Source: CAD feature listing. Evaluate the final solid. Frame: model axes, mm. A direction names the side the tool comes from. Give positions to 0.01 mm unless a question says otherwise; leave off trailing zeros. Loops run counter-clockwise (first coordinate to the right, second up) from the corner with the lowest first, then second, coordinate; pieces in that order, holes last. Notation, with made-up numbers: M -12,45 L 10,45 A10 ccw 10,64 Z; hole C 34,-5 d11. An arc over 180 degrees is marked long. Put each result on its own line as item: value.
from build123d import *

# Parameters (mm, degrees)
SKETCH1_R           = 5.969
SKETCH1_R_2         = 4.572
BASE_EXTRUDE_DEPTH  = 13.97
BOSS_EXTRUDE1_DEPTH = 7.112
SKETCH3_W           = 4.826
SKETCH3_H           = 3.048
CUT_EXTRUDE1_DEPTH  = 1.524
CUT_EXTRUDE2_START  = -6.605477
SKETCH4_W           = 1.524
SKETCH4_H           = 4.064
CUT_EXTRUDE2_DEPTH  = 6.605477
CUT_EXTRUDE3_REACH  = 10.382
SKETCH5_R           = 0.8001
BOSS_EXTRUDE2_DEPTH = 1.524
SKETCH7_R           = 0.508
CUT_EXTRUDE4_DEPTH  = 10.144
BOSS_EXTRUDE3_DEPTH = 1.524
BOSS_EXTRUDE4_START = -3.048
BOSS_EXTRUDE4_DEPTH = 3.048
CUT_EXTRUDE5_START  = -1.1176
CUT_EXTRUDE5_DEPTH  = 1.1176
CUT_EXTRUDE6_DEPTH  = 4.064


with BuildPart() as part:
    # Sketch1 → Base-Extrude (new body)
    with BuildSketch(Plane.XY):
        Circle(SKETCH1_R)
        Circle(SKETCH1_R_2, mode=Mode.SUBTRACT)
    extrude(amount=BASE_EXTRUDE_DEPTH)

    # Sketch2 → Boss-Extrude1 (add)
    with BuildSketch(Plane.XY.offset(13.5636)):
        with BuildLine():
            Line((-2.413, -5.459523056), (-3.937, -8.763))
            Line((-3.937, -8.763), (-3.937, -12.065))
            Line((-3.937, -12.065), (-2.413, -12.065))
            Line((-2.413, -12.065), (-2.413, -15.113))
            Line((-2.413, -15.113), (2.413, -15.113))
            Line((2.413, -15.113), (2.413, -12.065))
            Line((2.413, -12.065), (3.937, -12.065))
            Line((3.937, -12.065), (3.937, -8.763))
            Line((3.937, -8.763), (2.413, -5.459523056))
            ThreePointArc((2.413, -5.459523056), (0, -5.969), (-2.413, -5.459523056))
        make_face()
    extrude(amount=-BOSS_EXTRUDE1_DEPTH)

    # Sketch3 → Cut-Extrude1 (cut)
    with BuildSketch(Plane.XY.offset(13.97)):
        with Locations((0, -13.589)):
            Rectangle(SKETCH3_W, SKETCH3_H)
    extrude(amount=-CUT_EXTRUDE1_DEPTH, mode=Mode.SUBTRACT)

    # Sketch4 → Cut-Extrude2 (cut)
    with BuildSketch(Plane.XZ.offset(12.065).offset(CUT_EXTRUDE2_START)):
        with Locations((3.175, 8.4836)):
            Rectangle(SKETCH4_W, SKETCH4_H)
        with Locations((-3.175, 8.4836)):
            Rectangle(SKETCH4_W, SKETCH4_H)
    extrude(amount=CUT_EXTRUDE2_DEPTH, mode=Mode.SUBTRACT)

    # Sketch5 → Cut-Extrude3 (cut, up to next)
    with BuildSketch(Plane(origin=(2.413, 0, 0), x_dir=(0, 0, -1), z_dir=(1, 0, 0)), mode=Mode.PRIVATE) as cut_extrude3_sk1:
        with Locations((-9.7155, -10.577465123)):
            Circle(SKETCH5_R)
    cut_extrude3_tool1 = extrude(cut_extrude3_sk1.sketch, amount=-CUT_EXTRUDE3_REACH, mode=Mode.PRIVATE) & part.part
    add(cut_extrude3_tool1.solids().sort_by_distance((2.413, -10.577465, 9.7155))[0], mode=Mode.SUBTRACT)

    # Sketch6 → Boss-Extrude2 (add)
    with BuildSketch(Plane.XY.offset(9.144)):
        with BuildLine():
            Line((-2.794, 5.274706153), (-1.524, 12.451775059))
            ThreePointArc((-1.524, 12.451775059), (-1.263283995, 12.902874385), (-0.773656889, 13.081))
            Line((-0.773656889, 13.081), (0.773656889, 13.081))
            ThreePointArc((0.773656889, 13.081), (1.263283995, 12.902874385), (1.524, 12.451775059))
            Line((1.524, 12.451775059), (2.794, 5.274706153))
            ThreePointArc((2.794, 5.274706153), (0, 5.969), (-2.794, 5.274706153))
        make_face()
    extrude(amount=-BOSS_EXTRUDE2_DEPTH)

    # Sketch7 → Cut-Extrude4 (cut, through all)
    with BuildSketch(Plane.XY.offset(9.144)):
        with Locations((0, 11.811)):
            Circle(SKETCH7_R)
    extrude(amount=-CUT_EXTRUDE4_DEPTH, mode=Mode.SUBTRACT)

    # Sketch8 → Boss-Extrude3 (add)
    with BuildSketch(Plane(origin=(0, 0, 0), x_dir=(-1, 0, 0), z_dir=(0, 0, -1))):
        with BuildLine():
            Line((-1.016, 4.873623966), (-1.016, 5.881896378))
            ThreePointArc((-1.016, 5.881896378), (0, 5.969), (1.016, 5.881896378))
            Line((1.016, 5.881896378), (1.016, 4.873623966))
            ThreePointArc((1.016, 4.873623966), (0, 4.9784), (-1.016, 4.873623966))
        make_face()
    extrude(amount=BOSS_EXTRUDE3_DEPTH)

    # Sketch9 → Boss-Extrude4 (add)
    with BuildSketch(Plane.XZ.offset(15.113).offset(BOSS_EXTRUDE4_START)):
        Polygon((2.413, 9.4996), (2.9718, 8.7376), (2.9718, 7.2136), (2.413, 6.4516), align=None)
        Polygon((-2.413, 9.4996), (-2.9718, 8.7376), (-2.9718, 7.2136), (-2.413, 6.4516), align=None)
    extrude(amount=BOSS_EXTRUDE4_DEPTH)

    # Sketch10 → Cut-Extrude5 (cut)
    with BuildSketch(Plane.XY.offset(13.5636).offset(CUT_EXTRUDE5_START)):
        with BuildLine():
            Line((-2.413, -12.065), (2.413, -12.065))
            Line((2.413, -12.065), (2.413, -9.097590664))
            Line((2.413, -9.097590664), (0.935640411, -5.895213145))
            ThreePointArc((0.935640411, -5.895213145), (0, -5.969), (-0.935640411, -5.895213145))
            Line((-0.935640411, -5.895213145), (-2.413, -9.097590664))
            Line((-2.413, -9.097590664), (-2.413, -12.065))
        make_face()
    extrude(amount=CUT_EXTRUDE5_DEPTH, mode=Mode.SUBTRACT)

    # Sketch12 → Cut-Extrude6 (cut)
    with BuildSketch(Plane.XY.offset(12.446)):
        with BuildLine():
            Line((0.935640411, -5.895213145), (0.935640411, -9.777365123))
            Line((0.935640411, -9.777365123), (2.413, -9.777365123))
            Line((2.413, -9.777365123), (2.413, -11.377565123))
            Line((2.413, -11.377565123), (0.935640411, -11.377565123))
            Line((0.935640411, -11.377565123), (0.935640411, -13.589))
            Line((0.935640411, -13.589), (-0.935640411, -13.589))
            Line((-0.935640411, -13.589), (-0.935640411, -11.377565123))
            Line((-0.935640411, -11.377565123), (-2.413, -11.377565123))
            Line((-2.413, -11.377565123), (-2.413, -9.777365123))
            Line((-2.413, -9.777365123), (-0.935640411, -9.777365123))
            Line((-0.935640411, -9.777365123), (-0.935640411, -5.895213145))
            ThreePointArc((-0.935640411, -5.895213145), (0, -5.969), (0.935640411, -5.895213145))
        make_face()
    extrude(amount=-CUT_EXTRUDE6_DEPTH, mode=Mode.SUBTRACT)


solid = part.part
1. Section query D-D (z = 2.75). Output: boundary loops of the cut face in (x, y), plus the area to 3 significant figures.
Found:
outline: C 0,0 d11.94; hole C 0,0 d9.14
area: 46.3 mm^2
2. Draft query along X for faces 4 (the flat face through (2.972, -14, 8)), 5 (the flat face through (-0.936, -8, 10)), 6 (the flat face through (-2.972, -14, 8)), 7 (the flat face through (0, -10, 6.452)). Return one class per face: pulls with the +X half, pulls with the -X half, needs draft (parallel to the pull), parting line crosses it, or undercut.
Found:
face 4: pulls with the +X half
face 5: undercut
face 6: pulls with the -X half
face 7: needs draft
3. Section query C-C (z = 12). Output: boundary loops of the cut face in (x, y) (3 decimals), plus the area to 3 significant figures.
Found:
outline: M -3.937,-12.065 L -2.413,-12.065 L -2.413,-15.113 L 2.413,-15.113 L 2.413,-12.065 L 3.937,-12.065 L 3.937,-8.763 L 2.413,-5.46 A5.969 ccw long -2.413,-5.46 L -3.937,-8.763 Z; hole C 0,0 d9.144; hole M -2.413,-11.378 L -0.936,-11.378 L -0.936,-13.589 L 0.936,-13.589 L 0.936,-11.378 L 2.413,-11.378 L 2.413,-9.777 L 0.936,-9.777 L 0.936,-5.895 A5.969 cw -0.936,-5.895 L -0.936,-9.777 L -2.413,-9.777 Z
area: 87.3 mm^2
4. Access query for faces 1 (the flat face through (0.936, -12, 10)), 2 (the cylindrical face through (-0.01, 4.98, -0.75)), 3 (the flat face through (3.937, -10, 12)). Directions: +Z, -Z, +X, -X, +Y, -Y. A direction counts if a zero-diameter tool reaches every point of the face in a straight line with its end or side. Return the directions, or none.
Found:
face 1: +Z
face 2: -Z, -Y
face 3: +Z, -Z, +X, -Y
5. Section query A-A (x = 0). Output: boundary loops of the cut face in (y, z).
Found:
outline: M -15.11,6.45 L -5.97,6.45 L -5.97,0 L -4.57,0 L -4.57,13.97 L -5.97,13.97 L -5.97,8.38 L -13.59,8.38 L -13.59,12.45 L -15.11,12.45 Z; M 4.57,0 L 4.98,0 L 4.98,-1.52 L 5.97,-1.52 L 5.97,7.62 L 11.3,7.62 L 11.3,9.14 L 5.97,9.14 L 5.97,13.97 L 4.57,13.97 Z; M 12.32,7.62 L 13.08,7.62 L 13.08,9.14 L 12.32,9.14 Z
6. Contact query for flat-ended pins moving along their axis: P1, Ø1.5, axis at x = 3, y = -10, coming from the -Z side; P2, Ø1.5, axis at x = 0, z = 9.5, coming from the +Y side; P3, Ø5, axis at y = -10, z = 9, coming from the +X side; P4, Ø3, axis at y = -7, z = 11, coming from the +X side. Output: stop coordinate, or through.
Found:
P1: z = 6.45
P2: y = 13.08
P3: x = 3.94
P4: x = 3.82
7. Material intervals for line 1 (Y direction, x = 0, z = 8.65); line 2 (X direction, y = -12.25, z = 12.25); line 3 (X direction, y = -0.25, z = 5.25), sorted ascending. Write a range as from..to.
Found:
line 1: -15.11..-13.59, -5.97..-4.57, 4.57..11.3, 12.32..13.08
line 2: -2.41..-0.94, 0.94..2.41
line 3: -5.96..-4.57, 4.57..5.96
8. Section query B-B (y = 0). Output: boundary loops of the cut face in (x, z).
Found:
outline: M -5.97,0 L -4.57,0 L -4.57,13.97 L -5.97,13.97 Z; M 4.57,0 L 5.97,0 L 5.97,13.97 L 4.57,13.97 Z
